Here's how the part is built. I have some questions about the finished solid (model axes, mm). A direction names the side the tool comes from. Coordinates: 2 decimals unless noted, no trailing zeros. Write each loop counter-clockwise with the first axis right and the second up, starting at its lowest first coordinate (ties: lowest second). Pieces come first, ordered by that corner, then holes.
```python
from build123d import *

# Parameters (mm, degrees)
DODANIE_WYCI_GNI_CIE1_DEPTH = 20
SZKIC1_R                    = 32.5
SZKIC1_R_2                  = 22.5
DODANIE_WYCI_GNI_CIE2_DEPTH = 40
DODANIE_WYCI_GNI_CIE3_DEPTH = 20


with BuildPart() as part:
    # Szkic3 → Dodanie-wyciągnięcie1 (new body)
    with BuildSketch(Plane(origin=(0, 0, 0), x_dir=(1, 0, 0), z_dir=(0, 1, 0))):
        with BuildLine():
            Line((4.860466255, 32.134496539), (95.747764039, 18.387443016))
            ThreePointArc((95.747764039, 18.387443016), (98.790700476, 16.704132859), (100, 13.443674318))
            Line((100, 13.443674318), (100, 7.5))
            Line((100, 7.5), (68, 7.5))
            ThreePointArc((68, 7.5), (60.5, 0), (68, -7.5))
            Line((68, -7.5), (100, -7.5))
            Line((100, -7.5), (100, -12.976912833))
            ThreePointArc((100, -12.976912833), (98.79887335, -16.227845203), (95.772575492, -17.91686497))
            Line((95.772575492, -17.91686497), (5.021740697, -32.109688886))
            ThreePointArc((5.021740697, -32.109688886), (32.499897597, 0.081585638), (4.860466255, 32.134496539))
        make_face()
    extrude(amount=DODANIE_WYCI_GNI_CIE1_DEPTH)

    # Szkic1 → Dodanie-wyciągnięcie2 (add)
    with BuildSketch(Plane(origin=(0, 0, 0), x_dir=(1, 0, 0), z_dir=(0, 1, 0))):
        with Locations(Location((0, 0, 0), (0, 0, 81.398987984))):
            Circle(SZKIC1_R)
        with Locations(Location((0, 0, 0), (0, 0, 270))):
            Circle(SZKIC1_R_2, mode=Mode.SUBTRACT)
    extrude(amount=DODANIE_WYCI_GNI_CIE2_DEPTH)

    # Szkic2 → Dodanie-wyciągnięcie3 (add)
    with BuildSketch(Plane(origin=(0, 0, 0), x_dir=(1, 0, 0), z_dir=(0, 1, 0))):
        with BuildLine():
            Line((-28.831406487, 15), (-55, 15))
            Line((-55, 15), (-55, -15))
            Line((-55, -15), (-28.831406487, -15))
            ThreePointArc((-28.831406487, -15), (-32.5, 0), (-28.831406487, 15))
        make_face()
    extrude(amount=DODANIE_WYCI_GNI_CIE3_DEPTH)


solid = part.part
```
1) Imagine slicing it at B-B on x = 0. Please give me the cut outline in (y, z).
Values follow:
outline: (0, -32.5) - (40, -32.5) - (40, -22.5) - (0, -22.5) - close; (0, 22.5) - (40, 22.5) - (40, 32.5) - (0, 32.5) - close
2) On a 3-axis mill with a long thin cutter (end or side, diameter ignored), from which of +Z, -Z, +X, -X, +Y, -Y can I reach the whole of each face in a straight line? I mean faces 4 (the face through (84, 10, -7.5)), 5 (the face through (-42, 10, 15)), 6 (the face through (-32.494, 24.164, -0.636)). Say none if no direction works.
Values follow:
face 4: +X, +Y, -Y
face 5: +Z, -X, +Y, -Y
face 6: +Y
3) Imagine slicing it at A-A on y = 15. Please give me the cut outline in (x, z), then the cut area to 3 significant figures.
Values follow:
outline: (-55, -15) - (-28.83, -15) arc R32.5 ccw to (4.86, -32.13) - (95.75, -18.39) arc R5 ccw to (100, -13.44) - (100, -7.5) - (68, -7.5) arc R7.5 cw to (68, 7.5) - (100, 7.5) - (100, 12.98) arc R5 ccw to (95.77, 17.92) - (5.02, 32.11) arc R32.5 ccw to (-28.83, 15) - (-55, 15) - close; hole circle Ø45 at (0, 0)
area: 5,240 mm2
4) Imagine slicing it at D-D on z = -28. Please give me the cut outline in (x, y).
Values follow:
outline: (-16.5, 0) - (32.2, 0) - (32.2, 20) - (16.5, 20) - (16.5, 40) - (-16.5, 40) - close
5) Will these pins go through, and if not, where does the flat tip stop? pin 1 (2 mm diameter, centred on x = 19.5, y = 33.5, fed in from +Z); pin 2 (1 mm diameter, centred on x = 45, z = 8.5, fed in from +Y); pin 3 (22 mm diameter, centred on x = 82.5, y = 7.5, fed in from +Z).
Values follow:
pin 1: stops at z = 26.72
pin 2: stops at y = 20
pin 3: stops at z = 21.71
6) I need wall thicknesses on probe 1 along X at (y, z) = (21, 0); probe 2 along Y at (x, z) = (86.5, -16.5); probe 3 along X at (y, z) = (29.5, 7). Which ranges of each line are inside material? Lowest first, please.
Values follow:
probe 1: x = -32.5 to -22.5, 22.5 to 32.5
probe 2: y = 0 to 20
probe 3: x = -31.74 to -21.38, 21.38 to 31.74
7) Imagine slicing it at C-C on z = 0. Please give me the cut outline in (x, y), then the cut area to 3 significant figures.
Values follow:
outline: (-55, 0) - (-22.5, 0) - (-22.5, 40) - (-32.5, 40) - (-32.5, 20) - (-55, 20) - close; (22.5, 0) - (60.5, 0) - (60.5, 20) - (32.5, 20) - (32.5, 40) - (22.5, 40) - close
area: 1,810 mm2
8) We'd pull the mould along Z, two halves only. Please class faces 1 (the face through (-42, 20, 0)), 2 (the face through (84, 10, 7.5)), 3 (the face through (98.76, 9.86, -16.74)): pulls with the +Z half, pulls with the -Z half, needs draft (parallel to the pull), parting line crosses it, or undercut.
Values follow:
face 1: needs draft
face 2: undercut
face 3: pulls with the -Z half
